```python
from build123d import *

# Parameters (mm, degrees)
SKETCH3_W           = 200
SKETCH3_H           = 200
BOSS_EXTRUDE1_DEPTH = 3
SKETCH4_R           = 1.5
SKETCH4_R_2         = 60
CUT_EXTRUDE1_DEPTH  = 5


with BuildPart() as part:
    # Sketch3 → Boss-Extrude1 (new body)
    with BuildSketch(Plane(origin=(0, 0, 0), x_dir=(1, 0, 0), z_dir=(0, 1, 0))):
        Rectangle(SKETCH3_W, SKETCH3_H)
    extrude(amount=BOSS_EXTRUDE1_DEPTH)

    # Sketch4 → Cut-Extrude1 (cut)
    with BuildSketch(Plane(origin=(0, 3, 0), x_dir=(1, 0, 0), z_dir=(0, 1, 0))):
        with Locations(Location((92, 92, 0), (0, 0, 270))):
            Circle(SKETCH4_R)
        with Locations(Location((92, -92, 0), (0, 0, 270))):
            Circle(SKETCH4_R)
        with Locations(Location((-92, -92, 0), (0, 0, 270))):
            Circle(SKETCH4_R)
        with Locations(Location((-92, 92, 0), (0, 0, 270))):
            Circle(SKETCH4_R)
        with Locations(Location((92, -25, 0), (0, 0, 270))):
            Circle(SKETCH4_R)
        with Locations(Location((17, -93, 0), (0, 0, 270))):
            Circle(SKETCH4_R)
        with Locations(Location((29, -73, 0), (0, 0, 270))):
            Circle(SKETCH4_R)
        with Locations(Location((75, 92, 0), (0, 0, 270))):
            Circle(SKETCH4_R)
        with Locations(Location((29, -27, 0), (0, 0, 270))):
            Circle(SKETCH4_R)
        with Locations(Location((17, -7, 0), (0, 0, 270))):
            Circle(SKETCH4_R)
        with Locations(Location((-92, -25, 0), (0, 0, 270))):
            Circle(SKETCH4_R)
        with Locations(Location((-17, -93, 0), (0, 0, 270))):
            Circle(SKETCH4_R)
        with Locations(Location((-29, -73, 0), (0, 0, 270))):
            Circle(SKETCH4_R)
        with Locations(Location((-29, -27, 0), (0, 0, 270))):
            Circle(SKETCH4_R)
        with Locations(Location((-17, -7, 0), (0, 0, 270))):
            Circle(SKETCH4_R)
        with Locations((0, 100)):
            Circle(SKETCH4_R_2)
        with Locations(Location((-75, 92, 0), (0, 0, 270))):
            Circle(SKETCH4_R)
        with Locations(Location((0, 0, 0), (0, 0, 270))):
            Circle(SKETCH4_R)
    extrude(amount=-CUT_EXTRUDE1_DEPTH, mode=Mode.SUBTRACT)


solid = part.part
```
Here's how the part is built. I have some questions about the finished solid (model axes, mm). Coordinates: 2 decimals unless noted, no trailing zeros. Loops run counter-clockwise (first coordinate to the right, second up) from the corner with the lowest first, then second, coordinate; pieces in that order, holes last. Notation, with made-up numbers: (87.5, 17) - (95.5, 17) arc R17 cw to (95.5, 31) - close; hole circle Ø5 at (33.5, 34). An arc over 180 degrees is marked (long way). Answer as CSV lines item,"result".
Q1. We'd pull the mould along X, two halves only. Please class faces 1 (the face through (-1.319, 1.521, -40.015)), 2 (the face through (-1, 3, 21)): pulls with the +X half, pulls with the -X half, needs draft (parallel to the pull), parting line crosses it, or undercut.
Response:
face 1,"undercut"
face 2,"needs draft"
Q2. For pin 1 (2.5 mm diameter, centred on x = -29, z = 73, fed in from +Y), with a flat end and sliding along its axis, tell me the tip position at first contact or that it passes through.
Response:
pin 1,"through"
Q3. If we section it at C-C, the plane x = -55.5: Write out the boundary of the cut face in (y, z), and give its area (3 significant figures).
Response:
outline,"(0, -77.2) - (3, -77.2) - (3, 100) - (0, 100) - close"
area,"532 mm2"
Q4. If I drill on L1, parallel to Z at x = 92, y = 1.2; L2, parallel to X at y = 0.7, z = 27; L3, parallel to X at y = 0.85, z = -92, over which ranges is the centre line in solid material (lowest first)? Write a range as [from, to].
Response:
L1,"[-100, -93.5], [-90.5, 23.5], [26.5, 90.5], [93.5, 100]"
L2,"[-100, -30.5], [-27.5, 27.5], [30.5, 100]"
L3,"[-100, -93.5], [-90.5, -76.5], [-73.5, -59.46], [59.46, 73.5], [76.5, 90.5], [93.5, 100]"
Q5. If we section it at B-B, the plane z = -61: Write out the boundary of the cut face in (x, y).
Response:
outline,"(-100, 0) - (-45.6, 0) - (-45.6, 3) - (-100, 3) - close; (45.6, 0) - (100, 0) - (100, 3) - (45.6, 3) - close"
Q6. If we section it at A-A, the plane y = 0.85: Give the number of separate pieces and of enclosed holes in the cut face, and give its area (3 significant figures).
Response:
separate pieces,"1"
enclosed holes,"17"
area,"34,200 mm2"
